Source: CAD feature listing. Evaluate the final solid. Frame: model axes, mm. A direction names the side the tool comes from. Coordinates: 2 decimals unless noted, no trailing zeros. Write each loop counter-clockwise with the first axis right and the second up, starting at its lowest first coordinate (ties: lowest second). Pieces come first, ordered by that corner, then holes. Notation, with made-up numbers: (18, -34.75) - (40, -34.75) arc R5 ccw to (40, -28.75) - close; hole circle Ø10 at (-24, -22.75). An arc over 180 degrees is marked (long way). One line per question, with ' | ' between items.
Autodesk Inventor part; units mm, degrees
ref_plane "YZ Plane" through (0, 0, 0) normal (1, 0, 0) x (0, 1, 0)
ref_plane "XZ Plane" through (0, 0, 0) normal (0, 1, 0) x (-1, 0, 0)
ref_plane "XY Plane" through (0, 0, 0) normal (0, 0, 1) x (1, 0, 0)
sketch "Sketch1" plane through (0, 0, 0) normal (0, 1, 0) x (-1, 0, 0)
  line L0 (0, 0) -> (1.6, 0)
  line L1 (1.6, -41.2616) -> (0, -41.2616)
  line L2 (0, -41.2616) -> (0, 0)
  line L3 (1.6, -0.8) -> (1.2, -0.8)
  line L4 (1.2, -0.8) -> (1.2, -1.2)
  line L5 (1.2, -1.2) -> (1.6, -1.2)
  line L6 (1.6, -14.1616) -> (1.2, -14.1616)
  line L7 (1.2, -14.1616) -> (1.2, -14.5616)
  line L8 (1.2, -14.5616) -> (1.6, -14.5616)
  line L9 (1.6, -35.5616) -> (1.5, -35.5616)
  line L10 (1.5, -35.5616) -> (1.5, -41.2616)
  line L11 (1.5, -41.2616) -> (1.6, -41.2616)
  line L12 (1.6, -14.5616) -> (1.6, -35.5616)
  line L13 (1.6, 0) -> (1.6, -0.8)
  line L14 (1.6, -1.2) -> (1.6, -14.1616)
  dimension "d0" = 5.7
  dimension "d1" = 21.4
  dimension "d2" = 0.8
  dimension "d3" = 0.4
  dimension "d4" = 1.2
  dimension "d6" = 0.4
  dimension "d7" = 1.5
revolve "Revolution1" add sketch "Sketch1" angle 360 about axis through (0, 0, -41.2616) along (0, 0, 1)
thread "Thread1"
properties part number "500-104" material "Steel"
Item 1: Pin query (flat end, axial travel): pin 1 Ø1 at (y, z) = (-1, -29) entering from -X. Return the tip coordinate at first contact, or that it passes through.
Check sheet entries:
pin 1: x = -1.52
Item 2: Access query for faces 5 (the face through (1.5, 0.07, -38.45)), 6 (the face through (-1, -1, -1.2)), 7 (the face through (1.27, -0.97, -25.21)). Directions: +Z, -Z, +X, -X, +Y, -Y. A direction counts if a zero-diameter tool reaches every point of the face in a straight line with its end or side. Return the directions, or none.
Check sheet entries:
face 5: -Z | face 6: none | face 7: +Z, -Z
Item 3: Cut plane B-B on y = 0.75. Return loops of the section in (x, z).
Check sheet entries:
outline: (-1.41, -35.56) - (-1.3, -35.56) - (-1.3, -41.26) - (1.3, -41.26) - (1.3, -35.56) - (1.41, -35.56) - (1.41, -14.56) - (0.94, -14.56) - (0.94, -14.16) - (1.41, -14.16) - (1.41, -1.2) - (0.94, -1.2) - (0.94, -0.8) - (1.41, -0.8) - (1.41, 0) - (-1.41, 0) - (-1.41, -0.8) - (-0.94, -0.8) - (-0.94, -1.2) - (-1.41, -1.2) - (-1.41, -14.16) - (-0.94, -14.16) - (-0.94, -14.56) - (-1.41, -14.56) - close
Item 4: Ray query, line 1 along Z through (x, y) = (0.4, 1.2); line 2 along X through (y, z) = (1.05, -29); line 3 along Y through (x, z) = (0.9, -37.5). Return the intervals inside material, ascending. Write a range as [from, to].
Check sheet entries:
line 1: [-41.26, -14.56], [-14.16, -1.2], [-0.8, 0] | line 2: [-1.21, 1.21] | line 3: [-1.2, 1.2]
Item 5: Mould query, pull axis Z, two halves, no side actions, for faces 1 (the face through (0, 0, -41.262)), 2 (the face through (0, 0, 0)), 3 (the face through (-1, -1, -0.8)), 4 (the face through (1.27, -0.97, -7.77)). Classes: pulls with the +Z half, pulls with the -Z half, needs draft (parallel to the pull), parting line crosses it, or undercut.
Check sheet entries:
face 1: pulls with the -Z half | face 2: pulls with the +Z half | face 3: undercut | face 4: needs draft
Item 6: Cut plane C-C on x = 0.8. Return loops of the section in (y, z).
Check sheet entries:
outline: (-1.39, -35.56) - (-1.27, -35.56) - (-1.27, -41.26) - (1.27, -41.26) - (1.27, -35.56) - (1.39, -35.56) - (1.39, -14.56) - (0.89, -14.56) - (0.89, -14.16) - (1.39, -14.16) - (1.39, -1.2) - (0.89, -1.2) - (0.89, -0.8) - (1.39, -0.8) - (1.39, 0) - (-1.39, 0) - (-1.39, -0.8) - (-0.89, -0.8) - (-0.89, -1.2) - (-1.39, -1.2) - (-1.39, -14.16) - (-0.89, -14.16) - (-0.89, -14.56) - (-1.39, -14.56) - close
Item 7: Cut plane A-A on z = -30. Return loops of the section in (x, y), and give its area (3 significant figures).
Check sheet entries:
outline: circle Ø3.2 at (0, 0) | area: 8.04 mm²
